from build123d import *

# Parameters (mm, degrees)
SKETCH2_R                = 14
SKETCH2_R_2              = 1.75
SKETCH2_R_3              = 7.5
FLANGE_DEPTH             = 2
SKETCH3_R                = 8.5
O_RING_SEAT_DEPTH        = 0.5
BOSS_EXTRUDE1_START      = 10
SKETCH4_R                = 9.5
SKETCH4_R_2              = 7.5
BOSS_EXTRUDE1_DEPTH      = 10
SKETCH5_R                = 1
OUTLET_DEPTH             = 24.151673806
BOSS_EXTRUDE2_REACH      = 31.871
BOSS_EXTRUDE2_END_RADIUS = 9.5
SKETCH6_R                = 3
SKETCH6_R_2              = 1


with BuildPart() as part:
    # Sketch2 → Flange (new body)
    with BuildSketch(Plane(origin=(0, 0, 0), x_dir=(0, 0, -1), z_dir=(1, 0, 0))):
        Circle(SKETCH2_R)
        with Locations((0, 12)):
            Circle(SKETCH2_R_2, mode=Mode.SUBTRACT)
        with Locations((12, 0)):
            Circle(SKETCH2_R_2, mode=Mode.SUBTRACT)
        with Locations((0, -12)):
            Circle(SKETCH2_R_2, mode=Mode.SUBTRACT)
        with Locations((-12, 0)):
            Circle(SKETCH2_R_2, mode=Mode.SUBTRACT)
        Circle(SKETCH2_R_3, mode=Mode.SUBTRACT)
    flange = extrude(amount=-FLANGE_DEPTH)

    # Sketch3 → O-Ring Seat (cut)
    with BuildSketch(Plane.ZY.offset(2)):
        Circle(SKETCH3_R)
    o_ring_seat = extrude(amount=-O_RING_SEAT_DEPTH, mode=Mode.SUBTRACT)

    # Sketch4 → Boss-Extrude1 (add)
    with BuildSketch(Plane(origin=(0, 0, 0), x_dir=(0, 0, -1), z_dir=(1, 0, 0)).offset(BOSS_EXTRUDE1_START)):
        Circle(SKETCH4_R)
        Circle(SKETCH4_R_2, mode=Mode.SUBTRACT)
    extrude(amount=-BOSS_EXTRUDE1_DEPTH)

    # Mirror1: Flange, O-Ring Seat across plane
    add(flange.mirror(Plane(origin=(5, 0, 0), x_dir=(0, 0, 1), z_dir=(1, 0, 0))))
    add(o_ring_seat.mirror(Plane(origin=(5, 0, 0), x_dir=(0, 0, 1), z_dir=(1, 0, 0))), mode=Mode.SUBTRACT)

    # Sketch5 → Outlet (cut, through all)
    with BuildSketch(Plane(origin=(0, 0, 0), x_dir=(1, 0, 0), z_dir=(0, 1, 0))):
        with Locations(Location((5, 6.5, 0), (0, 0, 90))):
            Circle(SKETCH5_R)
    outlet = extrude(amount=OUTLET_DEPTH, mode=Mode.SUBTRACT)

    # Boss-Extrude2: up to this cylinder (the profile starts outside it)
    boss_extrude2_end = Plane(origin=(5, 0, 0), z_dir=(-1, 0, 0)) * Cylinder(BOSS_EXTRUDE2_END_RADIUS, 83.742, mode=Mode.PRIVATE)
    # Sketch6 → Boss-Extrude2 (add, up to the surface)
    with BuildSketch(Plane(origin=(0, 9.5, 0), x_dir=(1, 0, 0), z_dir=(0, 1, 0)), mode=Mode.PRIVATE) as boss_extrude2_sk1:
        with Locations(Location((5, 6.5, 0), (0, 0, 270))):
            Circle(SKETCH6_R)
        with Locations(Location((5, 6.5, 0), (0, 0, 90))):
            Circle(SKETCH6_R_2, mode=Mode.SUBTRACT)
    boss_extrude2_tool1 = extrude(boss_extrude2_sk1.sketch, amount=-BOSS_EXTRUDE2_REACH, mode=Mode.PRIVATE) - boss_extrude2_end
    boss_extrude2 = boss_extrude2_tool1.solids().sort_by_distance((5, 9.5, -9.415147))[0]
    add(boss_extrude2)

    # Inlet: Outlet, Boss-Extrude2 across plane
    add(outlet.mirror(Plane.XY), mode=Mode.SUBTRACT)
    add(boss_extrude2.mirror(Plane.XY))


solid = part.part
Check sheet for the modelled part. Datum: model origin and axes. Units: mm. A direction names the side the tool comes from. Give positions to 0.01 mm unless a question says otherwise; leave off trailing zeros. Write each loop counter-clockwise with the first axis right and the second up, starting at its lowest first coordinate (ties: lowest second). Pieces come first, ordered by that corner, then holes. Notation, with made-up numbers: (68.25, 24.5) -> (126.25, 24.5) arc R11 cw to (126.25, 32.5) -> close; hole circle Ø2 at (44, -6.5). An arc over 180 degrees is marked (long way). One line per item, written item: value. Start each with the question number.
Item 1: Section check B-B on x = 5. Record the cut outline in (y, z), then the cut area to 3 significant figures.
Item 2: Section check C-C on z = -6.5. State how many separate pieces and enclosed holes the cut face has, then the cut area to 3 significant figures.
Item 3: Draft check along X on faces 5 (the flat face through (10, -9.1, 3.3)), 6 (the cylindrical face through (-0.986, -5.362, -12.932)), 7 (the flat face through (12, -9, 0)). Enter one of: +X half, -X half, draft (parallel to the pull), parting line (faces both ways), or undercut.
Item 4: Section check A-A on y = 12. Record the cut outline in (x, z), then the cut area to 3 significant figures.
Item 5: Material ranges on probe 1 along Y at (x, z) = (10.7, 0); probe 2 along X at (y, z) = (8.3, 6.5); probe 3 along X at (y, z) = (12, -6), recorded low to high. Write a range as from..to.
Item 6: Tool access check on faces 1 (the flat face through (11.5, -8, 0)), 2 (the flat face through (5, 9.5, -5)), 3 (the cylindrical face through (-1.754, 7.167, 4.57)), 4 (the cylindrical face through (5.07, -9.274, 2.059)). Record the directions out of +Z, -Z, +X, -X, +Y, -Y that give a thin tool (end or side, any length) a straight path to the whole face; none if there is none.
Item 7: Gauge pin test, flat ends, axial feed: pin 1 (6.5 mm diameter, centred on x = 4.5, z = 7, fed in from +Y); pin 2 (14 mm diameter, centred on y = -1.5, z = 1, fed in from +X); pin 3 (5 mm diameter, centred on x = 4, y = -4, fed in from -Z); pin 4 (2 mm diameter, centred on x = 10, z = 10, fed in from +Y). Record the tip position at first contact, or that the pin passes through.
Item 8: Section check D-D on y = -2.25. Record the cut outline in (x, z), then the cut area to 3 significant figures.
Results list:
1. outline: (0, -9.5) -> (9.5, -9.5) -> (9.5, -7.5) -> (0, -7.5) arc R7.5 cw to (0, 7.5) -> (9.5, 7.5) -> (9.5, 9.5) -> (0, 9.5) arc R9.5 ccw to start; (5.1, -5.5) -> (9.5, -5.5) -> (9.5, -3.5) -> (8.83, -3.5) arc R9.5 ccw to (8.83, 3.5) -> (9.5, 3.5) -> (9.5, 5.5) -> (5.1, 5.5) arc R7.5 cw to start
1. area: 120 mm²
2. separate pieces: 3
2. enclosed holes: 0
2. area: 133 mm²
3. face 5: undercut
3. face 6: draft
3. face 7: +X half
4. outline: (-2, -7.21) -> (0, -7.21) -> (0, -1.75) -> (-2, -1.75) -> close; (-2, 1.75) -> (0, 1.75) -> (0, 7.21) -> (-2, 7.21) -> close; (10, -7.21) -> (12, -7.21) -> (12, -1.75) -> (10, -1.75) -> close; (10, 1.75) -> (12, 1.75) -> (12, 7.21) -> (10, 7.21) -> close
4. area: 43.7 mm²
5. probe 1: -14..-13.75, -10.25..-7.5, 7.5..10.25, 13.75..14
5. probe 2: -2..0, 2..4, 6..8, 10..12
5. probe 3: -2..0, 10..12
6. face 1: +X
6. face 2: +Z, -Z, +Y
6. face 3: -X
6. face 4: none
7. pin 1: y = 9.5
7. pin 2: x = 12
7. pin 3: z = -9.38
7. pin 4: y = 10.72
8. outline: (-2, -13.82) -> (0, -13.82) -> (0, -9.23) -> (10, -9.23) -> (10, -13.82) -> (12, -13.82) -> (12, -8.2) -> (11.5, -8.2) -> (11.5, -7.15) -> (-1.5, -7.15) -> (-1.5, -8.2) -> (-2, -8.2) -> close; (-2, 8.2) -> (-1.5, 8.2) -> (-1.5, 7.15) -> (11.5, 7.15) -> (11.5, 8.2) -> (12, 8.2) -> (12, 13.82) -> (10, 13.82) -> (10, 9.23) -> (0, 9.23) -> (0, 13.82) -> (-2, 13.82) -> close
8. area: 92.7 mm²
